Part model, mm, in its own coordinate system. Face numbers are marked on the shaded views. A direction names the side the tool comes from. Give positions to 0.01 mm unless a question says otherwise; leave off trailing zeros. Order: outer loops, then holes, each group sorted by start corner. A loop starts at its lowest first (then second) coordinate and runs counter-clockwise, first axis right, second up. Notation, with made-up numbers: (0.5, 61.25) - (59.5, 61.25) arc R17 ccw to (59.5, 76.25) - close; hole circle Ø6 at (79, 0.5). An arc over 180 degrees is marked (long way). One line per item, written item: value.
```python
from build123d import *

# Parameters (mm, degrees)
SKETCH1_R                  = 30
BOSS_EXTRUDE1_DEPTH        = 10
SKETCH2_R                  = 15
CUT_EXTRUDE1_DEPTH         = 10
CUT_EXTRUDE4_DEPTH         = 0.01
BOSS_EXTRUDE2_DEPTH        = 0.5
SKETCH9_R                  = 30
BOSS_EXTRUDE3_DEPTH        = 10
BOSS_EXTRUDE4_DEPTH        = 0.5
LPATTERN1_COUNT            = 2
LPATTERN1_PITCH            = 21
SKETCH11_R                 = 30
BOSS_EXTRUDE5_DEPTH        = 10
LPATTERN2_COUNT            = 2
LPATTERN2_PITCH            = 21
SKETCH12_R                 = 30
BOSS_EXTRUDE6_DEPTH        = 10
SKETCH13_W                 = 0.2
SKETCH13_H                 = 22
BOSS_EXTRUDE7_DEPTH        = 20.5
SKETCH14_W                 = 0.2
SKETCH14_H                 = 22
BOSS_EXTRUDE8_DEPTH        = 20.5
SKETCH15_R                 = 30
BOSS_EXTRUDE9_DEPTH        = 75
SKETCH16_R                 = 18
CUT_EXTRUDE5_DEPTH         = 2
SKETCH42_R                 = 29.95
BOSS_EXTRUDE10_DEPTH       = 25
SKETCH46_R                 = 19.95
BOSS_EXTRUDE11_DEPTH       = 15
CUT_EXTRUDE8_DEPTH         = 10
SKETCH48_R                 = 12
CUT_EXTRUDE9_DEPTH         = 3
SKETCH49_R                 = 9
BOSS_EXTRUDE12_DEPTH       = 2
CUT_EXTRUDE10_DEPTH        = 1
M20X1_5_TAPPED_HOLE1_D     = 18.5
M20X1_5_TAPPED_HOLE1_DEPTH = 34.5
M20X1_5_TAPPED_HOLE1_TIP   = 5.557960726


with BuildPart() as part:
    # Sketch1 → Boss-Extrude1 (new body)
    with BuildSketch(Plane(origin=(0, 0, 0), x_dir=(1, 0, 0), z_dir=(0, 1, 0))):
        with Locations(Location((0, 0, 0), (0, 0, 270))):  # turned: the seam where the file's is
            Circle(SKETCH1_R)
    extrude(amount=BOSS_EXTRUDE1_DEPTH)

    # Sketch2 → Cut-Extrude1 (cut)
    with BuildSketch(Plane.XZ):
        with Locations(Location((0, 0, 0), (0, 0, 270))):  # turned: the seam where the file's is
            Circle(SKETCH2_R)
    extrude(amount=-CUT_EXTRUDE1_DEPTH, mode=Mode.SUBTRACT)

    # Sketch7 → Cut-Extrude4 (cut)
    with BuildSketch(Plane(origin=(0, 10, 0), x_dir=(1, 0, 0), z_dir=(0, 1, 0))):
        Polygon((0, -23.5), (-0.5, -23.5), (-0.5, -22), (-2, -22), (-2, -21.5), (-0.5, -21.5), (-0.5, -20), (0, -20), (0, -21.5), (1.5, -21.5), (1.5, -22), (0, -22), align=None)
    extrude(amount=-CUT_EXTRUDE4_DEPTH, mode=Mode.SUBTRACT)

    # Sketch8 → Boss-Extrude2 (add)
    with BuildSketch(Plane(origin=(0, 10, 0), x_dir=(1, 0, 0), z_dir=(0, 1, 0))):
        with BuildLine():
            Line((27.915945712, 11), (43.415945712, 11))
            Line((43.415945712, 11), (43.415945712, -11))
            Line((43.415945712, -11), (27.915945712, -11))
            ThreePointArc((27.915945712, -11), (-30.005, 0), (27.915945712, 11))
        make_face()
    boss_extrude2 = extrude(amount=BOSS_EXTRUDE2_DEPTH)

    # Sketch9 → Boss-Extrude3 (add)
    with BuildSketch(Plane(origin=(0, 10.5, 0), x_dir=(1, 0, 0), z_dir=(0, 1, 0))):
        with Locations(Location((0, 0, 0), (0, 0, 270))):  # turned: the seam where the file's is
            Circle(SKETCH9_R)
    extrude(amount=BOSS_EXTRUDE3_DEPTH)

    # Sketch10 → Boss-Extrude4 (add)
    with BuildSketch(Plane(origin=(0, 20.5, 0), x_dir=(1, 0, 0), z_dir=(0, 1, 0))):
        with BuildLine():
            Line((-43.415945712, 11), (-27.915945712, 11))
            ThreePointArc((-27.915945712, 11), (30.005, 0), (-27.915945712, -11))
            Line((-27.915945712, -11), (-43.415945712, -11))
            Line((-43.415945712, -11), (-43.415945712, 11))
        make_face()
    boss_extrude4 = extrude(amount=BOSS_EXTRUDE4_DEPTH)

    # LPattern1: Boss-Extrude4 ×2
    with Locations(*[(0, -i * LPATTERN1_PITCH, 0) for i in range(1, LPATTERN1_COUNT)]):
        add(boss_extrude4)

    # Sketch11 → Boss-Extrude5 (add)
    with BuildSketch(Plane(origin=(0, 21, 0), x_dir=(1, 0, 0), z_dir=(0, 1, 0))):
        with Locations(Location((0, 0, 0), (0, 0, 270))):  # turned: the seam where the file's is
            Circle(SKETCH11_R)
    extrude(amount=BOSS_EXTRUDE5_DEPTH)

    # LPattern2: Boss-Extrude2 ×2
    with Locations(*[(0, i * LPATTERN2_PITCH, 0) for i in range(1, LPATTERN2_COUNT)]):
        add(boss_extrude2)

    # Sketch12 → Boss-Extrude6 (add)
    with BuildSketch(Plane(origin=(0, 31.5, 0), x_dir=(1, 0, 0), z_dir=(0, 1, 0))):
        with Locations(Location((0, 0, 0), (0, 0, 270))):  # turned: the seam where the file's is
            Circle(SKETCH12_R)
    extrude(amount=BOSS_EXTRUDE6_DEPTH)

    # Sketch13 → Boss-Extrude7 (add)
    with BuildSketch(Plane.XZ.offset(-31)):
        with Locations((43.315945712, 0)):
            Rectangle(SKETCH13_W, SKETCH13_H)
    extrude(amount=BOSS_EXTRUDE7_DEPTH)

    # Sketch14 → Boss-Extrude8 (add)
    with BuildSketch(Plane.XZ.offset(-20.5)):
        with Locations((-43.315945712, 0)):
            Rectangle(SKETCH14_W, SKETCH14_H)
    extrude(amount=BOSS_EXTRUDE8_DEPTH)

    # Sketch15 → Boss-Extrude9 (add)
    with BuildSketch(Plane.XZ.offset(0.5)):
        with Locations(Location((0, 0, 0), (0, 0, 90))):  # turned: the seam where the file's is
            Circle(SKETCH15_R)
    extrude(amount=BOSS_EXTRUDE9_DEPTH)

    # Sketch16 → Cut-Extrude5 (cut)
    with BuildSketch(Plane.XZ.offset(75.5)):
        with Locations(Location((0, 0, 0), (0, 0, 270))):  # turned: the seam where the file's is
            Circle(SKETCH16_R)
    extrude(amount=-CUT_EXTRUDE5_DEPTH, mode=Mode.SUBTRACT)

    # Sketch42 → Boss-Extrude10 (add)
    with BuildSketch(Plane(origin=(0, 41.5, 0), x_dir=(1, 0, 0), z_dir=(0, 1, 0))):
        with Locations(Location((0, 0, 0), (0, 0, 270))):  # turned: the seam where the file's is
            Circle(SKETCH42_R)
    extrude(amount=BOSS_EXTRUDE10_DEPTH)

    # Sketch45 → Revolve1 (revolve)
    with BuildSketch(Plane.XY, mode=Mode.PRIVATE) as revolve1_sk:
        Polygon((0, 66.5), (30, 66.5), (20, 74.5), (0, 74.5), align=None)
    revolve(revolve1_sk.sketch.rotate(Axis((0, 74.5, 0), (0, -1, 0)), 90), axis=Axis((0, 74.5, 0), (0, -1, 0)))  # turned: the seam where the file's is

    # Sketch46 → Boss-Extrude11 (add)
    with BuildSketch(Plane(origin=(0, 74.5, 0), x_dir=(1, 0, 0), z_dir=(0, 1, 0))):
        with Locations(Location((0, 0, 0), (0, 0, 180))):  # turned: the seam where the file's is
            Circle(SKETCH46_R)
    extrude(amount=BOSS_EXTRUDE11_DEPTH)

    # Sketch47 → Cut-Extrude8 (cut)
    with BuildSketch(Plane(origin=(0, 89.5, 0), x_dir=(1, 0, 0), z_dir=(0, 1, 0))):
        with BuildLine():
            Line((-15.922781257, 12.019464923), (15.922781257, 12.019464923))
            ThreePointArc((15.922781257, 12.019464923), (0, 19.95), (-15.922781257, 12.019464923))
        make_face()
        with BuildLine():
            Line((-15.922781257, -12.019464923), (15.922781257, -12.019464923))
            ThreePointArc((15.922781257, -12.019464923), (0, -19.95), (-15.922781257, -12.019464923))
        make_face()
    extrude(amount=-CUT_EXTRUDE8_DEPTH, mode=Mode.SUBTRACT)

    # Sketch48 → Cut-Extrude9 (cut)
    with BuildSketch(Plane(origin=(0, 89.5, 0), x_dir=(1, 0, 0), z_dir=(0, 1, 0))):
        with Locations(Location((0, 0, 0), (0, 0, 180))):  # turned: the seam where the file's is
            Circle(SKETCH48_R)
    extrude(amount=-CUT_EXTRUDE9_DEPTH, mode=Mode.SUBTRACT)

    # Sketch49 → Boss-Extrude12 (add)
    with BuildSketch(Plane(origin=(0, 86.5, 0), x_dir=(1, 0, 0), z_dir=(0, 1, 0))):
        with Locations(Location((0, 0, 0), (0, 0, 180))):  # turned: the seam where the file's is
            Circle(SKETCH49_R)
    extrude(amount=BOSS_EXTRUDE12_DEPTH)

    # Sketch50 → Cut-Extrude10 (cut)
    with BuildSketch(Plane.XY.offset(30)):
        with BuildLine():
            Line((-9.074878192, -50.5), (-9.074878192, -18.5))
            ThreePointArc((-9.074878192, -18.5), (0, -16.105614601), (9.074878192, -18.5))
            Line((9.074878192, -18.5), (9.074878192, -50.5))
            ThreePointArc((9.074878192, -50.5), (0, -52.894385399), (-9.074878192, -50.5))
        make_face()
    cut_extrude10 = extrude(amount=-CUT_EXTRUDE10_DEPTH, mode=Mode.SUBTRACT)

    # Mirror1: Cut-Extrude10 across plane
    add(cut_extrude10.mirror(Plane.XY), mode=Mode.SUBTRACT)

    # M20x1.5 Tapped Hole1
    with Locations(Plane(origin=(0, -73.5, 0), x_dir=(0, 0, -1), z_dir=(0, -1, 0))):
        with Locations((0, 0)):
            Hole(M20X1_5_TAPPED_HOLE1_D / 2, depth=M20X1_5_TAPPED_HOLE1_DEPTH)
            with Locations((0, 0, -(M20X1_5_TAPPED_HOLE1_DEPTH + M20X1_5_TAPPED_HOLE1_TIP / 2))):  # 118° drill point
                Cone(0, M20X1_5_TAPPED_HOLE1_D / 2, M20X1_5_TAPPED_HOLE1_TIP, mode=Mode.SUBTRACT)


solid = part.part
```
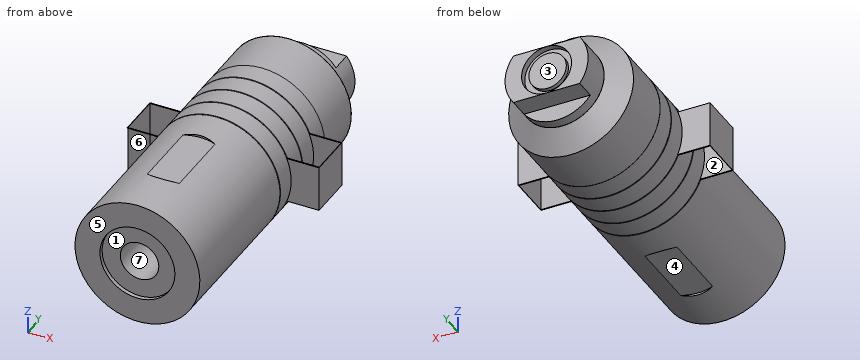
1) Which spindle directions (+Z, -Z, +X, -X, +Y, -Y) get a long thin tool onto all of the face, cutting with end or side? Do the marked faces 5, 6 and 7. Say none if no direction does.
Outcome:
face 5: +Z, -Z, +X, -X, -Y
face 6: +Z, -Z
face 7: -Y
2) Mould opens along Z. For the marked faces 1, 2, 3 and 4 say: released by +Z, released by -Z, zero draft, split by the parting line, or undercut.
Outcome:
face 1: undercut
face 2: zero draft
face 3: undercut
face 4: released by -Z
3) Drill centre lines: line 1 along X through (y, z) = (-74, 0); line 2 along X through (y, z) = (-56, 0). Where is each one in solid material? Low to high. Write a range as from..to.
Outcome:
line 1: x = -30..-18, 18..30
line 2: x = -30..-9.25, 9.25..30
4) Cut at A-A, the plane y = 17.5. Give the cut face in (x, z).
Outcome:
outline: (-43.42, -11) - (-43.22, -11) - (-43.22, 11) - (-43.42, 11) - close; circle Ø60 at (0, 0); (43.22, -11) - (43.42, -11) - (43.42, 11) - (43.22, 11) - close
5) Pin check, flat tips, straight feed: pin 1 (1.5 mm diameter, centred on y = 35, z = -14.5, fed in from +X); pin 2 (3 mm diameter, centred on y = -43, z = 9, fed in from +X); pin 3 (1 mm diameter, centred on x = 11.5, y = -38.5, fed in from +Z). Stop position of each tip, or through.
Outcome:
pin 1: stops at x = 26.66
pin 2: stops at x = 29.05
pin 3: stops at z = 27.91
